Design review of the part built by this model. Coordinates are the model's own, in mm. Face numbers are marked on the shaded views. A direction names the side the tool comes from. Give positions to 0.01 mm unless a question says otherwise; leave off trailing zeros. Write each loop counter-clockwise with the first axis right and the second up, starting at its lowest first coordinate (ties: lowest second). Pieces come first, ordered by that corner, then holes. Notation, with made-up numbers: M 19,22 L 38,22 A16 cw 38,32 Z; hole C 29,48.5 d9. An arc over 180 degrees is marked long. Write each question's results on one line, items separated by ' | '. Start each with the question number.
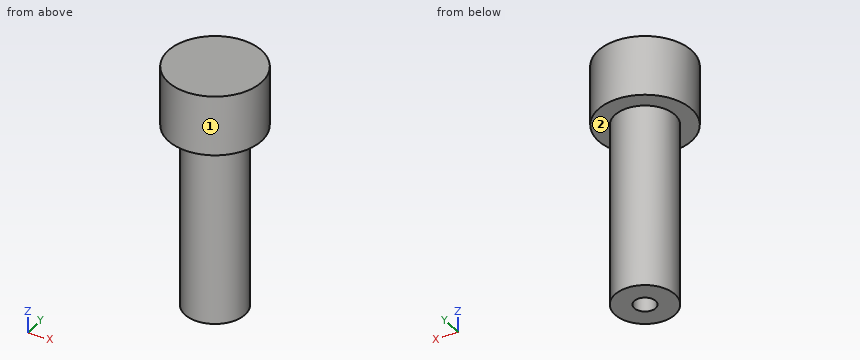
from build123d import *

# Parameters (mm, degrees)
F0_R     = 11.1125
F1_DEPTH = 7.1374
F2_R     = 7.1374
F3_DEPTH = 50.8
F4_R     = 2.5527
F5_DEPTH = 12.7


with BuildPart() as f1:
    # F0 (on Top) → F1 (new body, symmetric)
    with BuildSketch(Plane.XY):
        Circle(F0_R)
    extrude(amount=F1_DEPTH, both=True)

    # F2 (on Top) → F3 (join)
    with BuildSketch(Plane.XY):
        Circle(F2_R)
    extrude(amount=-F3_DEPTH)

    # F4 (on face) → F5 (cut)
    with BuildSketch(Plane(origin=(0, 0, -50.8), x_dir=(1, 0, 0), z_dir=(0, 0, -1))):
        Circle(F4_R)
    extrude(amount=-F5_DEPTH, mode=Mode.SUBTRACT)


solid = f1.part
Q1. For the marked faces 1 and 2, list the 3-axis set-ups (+Z, -Z, +X, -X, +Y, -Y) from which the entire face can be reached by the end or side of a thin tool; tool diameter is ignored.
Q2. Wall thickness on line 1 along Y through (x, z) = (0, -46); line 2 along Z through (x, y) = (1.75, -1); line 3 along Y through (x, z) = (0.25, -15.5): over which ranges is each line inside the solid? List them lowest first. Write a range as from..to.
Q3. We need section B-B on x = 0. Write out the cut boundary in (y, z), and give its area (3 significant figures).
Q4. We need section D-D on z = -26.5. Write out the cut boundary in (x, y).
Q5. For pin 1 Ø1.5 at (x, y) = (1, -0.5) entering from -Z; pin 2 Ø2 at (y, z) = (-6, -3.5) entering from +X; pin 3 Ø1.5 at (x, z) = (1, -27.5) entering from -Y, all flat-tipped, find the tip position at first contact; note any pin that passes through.
Q6. We need section A-A on z = -40. Write out the cut boundary in (x, y).
Answer sheet:
1) face 1: +Z, -Z | face 2: -Z
2) line 1: -7.14..-2.55, 2.55..7.14 | line 2: -38.1..7.14 | line 3: -7.13..7.13
3) outline: M -11.11,-7.14 L -7.14,-7.14 L -7.14,-50.8 L -2.55,-50.8 L -2.55,-38.1 L 2.55,-38.1 L 2.55,-50.8 L 7.14,-50.8 L 7.14,-7.14 L 11.11,-7.14 L 11.11,7.14 L -11.11,7.14 Z | area: 876 mm^2
4) outline: C 0,0 d14.27
5) pin 1: z = -38.1 | pin 2: x = 9.92 | pin 3: y = -7.13
6) outline: C 0,0 d14.27; hole C 0,0 d5.11
